Model file for the job. Use its own axes, mm. A direction names the side the tool comes from. Give positions to 0.01 mm unless a question says otherwise; leave off trailing zeros. Loops run counter-clockwise (first coordinate to the right, second up) from the corner with the lowest first, then second, coordinate; pieces in that order, holes last. Notation, with made-up numbers: M 17.25,4 L 69.25,4 A14 ccw 69.25,9 Z; hole C 51,84 d10. An arc over 180 degrees is marked long. Answer in a Markdown table with one row per item.
```python
from build123d import *

# Parameters (mm, degrees)
SKETCH_2_W               = 30
SKETCH_2_H               = 5
CUT_EXTRUDE_1_DEPTH      = 6
CUT_EXTRUDE_2_DEPTH      = 185.932420089
CUT_EXTRUDE_2_DEPTH_BACK = 185.932420089
SKETCH_3_R               = 7
PATTERN_CIRCULAR_1_COUNT = 2
CHAMFER_1_SIZE           = 2


with BuildPart() as part:
    # Эскиз1 → Повернуть1 (revolve)
    with BuildSketch(Plane.XY, mode=Mode.PRIVATE) as revolve_1_sk:
        Polygon((0, 0), (0, 20), (35, 20), (35, 25), (65, 25), (65, 30), (115, 30), (115, 20), (180, 20), (180, 0), align=None)
    revolve(revolve_1_sk.sketch.rotate(Axis((0, 0, 0), (-1, 0, 0)), 90), axis=Axis((0, 0, 0), (-1, 0, 0)))

    # Эскиз2 → Вырез-Вытянуть1 (cut, symmetric)
    with BuildSketch(Plane.XY):
        with Locations((150, 17.5)):
            Rectangle(SKETCH_2_W, SKETCH_2_H)
    extrude(amount=CUT_EXTRUDE_1_DEPTH, both=True, mode=Mode.SUBTRACT)

    # Эскиз3 → Вырез-Вытянуть2 (cut, two sides: drawn at the far end of the back side and taken through both)
    with BuildSketch(Plane.XY.offset(-CUT_EXTRUDE_2_DEPTH_BACK)):
        with Locations((17, 0)):
            Circle(SKETCH_3_R)
    extrude(amount=CUT_EXTRUDE_2_DEPTH + CUT_EXTRUDE_2_DEPTH_BACK, mode=Mode.SUBTRACT)

    # Эскиз4 → Диаметр отверстия Ø16.0 (20)1 (revolve, cut)
    with BuildSketch(Plane(origin=(90, 30, 0), x_dir=(0, 0, 1), z_dir=(1, 0, 0))):
        Polygon((0, 0), (0, 26.00860619), (10, 20), (10, 0), align=None)
    hole_wizard_16_0_20_1 = revolve(axis=Axis((90, 36.35, 0), (0, -1, 0)), mode=Mode.SUBTRACT)

    # Круговой массив1: Диаметр отверстия Ø16.0 (20)1 ×2 about axis
    pattern_circular_1_axis = Axis((0, 0, 0), (1, 0, 0))
    for i in range(1, PATTERN_CIRCULAR_1_COUNT):
        add(hole_wizard_16_0_20_1.rotate(pattern_circular_1_axis, i * 360 / PATTERN_CIRCULAR_1_COUNT), mode=Mode.SUBTRACT)

    # Фаска1
    chamfer_1_edges = [part.edges().sort_by_distance(p)[0] for p in [
        (0, 0, 20),
        (180, 0, 20),
        (115, 0, 30),
        (65, 0, 30),
    ]]
    chamfer(chamfer_1_edges, length=CHAMFER_1_SIZE)


solid = part.part
```
(1) Wall check: L1, parallel to X at y = 21, z = 0; L2, parallel to X at y = -18, z = 0; L3, parallel to Z at x = 90, y = 19.5. Give the ranges that are in metal, low to high.
Established:
| item | result |
|---|---|
| L1 | x = 35 to 80, 100 to 115 |
| L2 | x = 0 to 80, 100 to 180 |
| L3 | z = -22.8 to -10, 10 to 22.8 |
(2) Which spindle directions (+Z, -Z, +X, -X, +Y, -Y) get a long thin tool onto all of the face, cutting with end or side? Do faces 4 (the flat face through (165, 17, 0)), 5 (the cylindrical face through (80.085, -20.14, 1.302)), 6 (the flat face through (115, -19, 7)). Say none if no direction does.
Established:
| item | result |
|---|---|
| face 4 | +Y |
| face 5 | -Y |
| face 6 | +X |
(3) Mould opens along Z. For faces 1 (the flat face through (65, -23, -11)), 2 (the cylindrical face through (90.322, -9.011, -28.615)), 3 (the flat face through (150, 17, -6)) say: pulls with the +Z half, pulls with the -Z half, needs draft (parallel to the pull), parting line crosses it, or undercut.
Established:
| item | result |
|---|---|
| face 1 | needs draft |
| face 2 | parting line crosses it |
| face 3 | undercut |
(4) Saw through at A-A, the plane y = 0. Give the cut face in (x, z), and give its area (3 significant figures).
Established:
| item | result |
|---|---|
| outline | M 0,-18 L 2,-20 L 10,-20 L 10,20 L 2,20 L 0,18 Z; M 24,-20 L 35,-20 L 35,-25 L 65,-25 L 65,-28 L 67,-30 L 113,-30 L 115,-28 L 115,-20 L 178,-20 L 180,-18 L 180,18 L 178,20 L 115,20 L 115,28 L 113,30 L 67,30 L 65,28 L 65,25 L 35,25 L 35,20 L 24,20 Z |
| area | 7,920 mm2 |
(5) Saw through at B-B, the plane x = 17. Give the cut face in (y, z) (3 decimals).
Established:
| item | result |
|---|---|
| outline | M -7,-18.735 L -7,18.735 A20 ccw Z; M 7,-18.735 A20 ccw 7,18.735 Z |
(6) Flat gauge pins, fed straight in: P1, Ø5, axis at x = 125, y = 11.5, coming from the +Z side; P2, Ø4, axis at x = 56, y = -16.5, coming from the -Z side; P3, Ø6, axis at x = 53, z = -0.5, coming from the +Y side. Where does each tip first touch, or does it go through?
Established:
| item | result |
|---|---|
| P1 | stops at z = 17.86 |
| P2 | stops at z = -20.37 |
| P3 | stops at y = 25 |
